```python
from build123d import *

# Parameters (mm, degrees)
SKETCH_2_R      = 27.5
SKETCH_2_R_2    = 15
SKETCH_2_R_3    = 1.5
EXTRUDE_4_DEPTH = 2


with BuildPart() as part:
    # 草图2 → 凸台-拉伸4 (new body)
    with BuildSketch(Plane.XY):
        with Locations((139.999999999, 2e-09)):
            Circle(SKETCH_2_R)
        with Locations((139.999999999, 2e-09)):
            Circle(SKETCH_2_R_2, mode=Mode.SUBTRACT)
        with Locations((156.999999999, -16.999999998)):
            Circle(SKETCH_2_R_3, mode=Mode.SUBTRACT)
        with Locations((122.999999999, -16.999999998)):
            Circle(SKETCH_2_R_3, mode=Mode.SUBTRACT)
        with Locations((122.999999999, 17.000000002)):
            Circle(SKETCH_2_R_3, mode=Mode.SUBTRACT)
        with Locations((156.999999999, 17.000000002)):
            Circle(SKETCH_2_R_3, mode=Mode.SUBTRACT)
        with Locations((149.999999999, 17.320508077)):
            Circle(SKETCH_2_R_3, mode=Mode.SUBTRACT)
        with Locations((129.917171064, 19.639898968)):
            Circle(SKETCH_2_R_3, mode=Mode.SUBTRACT)
        with Locations((129.917171064, -19.639898965)):
            Circle(SKETCH_2_R_3, mode=Mode.SUBTRACT)
        with Locations((149.999999999, -17.320508074)):
            Circle(SKETCH_2_R_3, mode=Mode.SUBTRACT)
        with Locations((157.320508075, -9.999999999)):
            Circle(SKETCH_2_R_3, mode=Mode.SUBTRACT)
        with Locations((157.320508075, 10.000000001)):
            Circle(SKETCH_2_R_3, mode=Mode.SUBTRACT)
    extrude(amount=EXTRUDE_4_DEPTH)


solid = part.part
```
Work out the finished part from the listing and answer in its coordinate system (mm). Coordinates: 2 decimals unless noted, no trailing zeros. Loops run counter-clockwise (first coordinate to the right, second up) from the corner with the lowest first, then second, coordinate; pieces in that order, holes last.
1) Consider probe 1 along Y at (x, z) = (131, 1.85); probe 2 along Y at (x, z) = (150, 0.45); probe 3 along X at (y, z) = (-13, 0.6). Determine where each line is inside the solid, lowest interval first.
Results:
probe 1: y = -25.99 to -20.68, -18.6 to -12, 12 to 18.6, 20.68 to 25.99
probe 2: y = -25.62 to -18.82, -15.82 to -11.18, 11.18 to 15.82, 18.82 to 25.62
probe 3: x = 115.77 to 132.52, 147.48 to 164.23
2) Section B-B (y = 0) is taken. Give the vertices of the cut face in (x, z), plus the area to 3 significant figures.
Results:
outline: (112.5, 0) - (125, 0) - (125, 2) - (112.5, 2) - close; (155, 0) - (167.5, 0) - (167.5, 2) - (155, 2) - close
area: 50.0 mm2
3) For a pull along Y with two mould halves and no side action, classify faces 1 (the flat face through (152, -12, 2)), 2 (the cylindrical face through (151.386, -17.895, 0.986)), 3 (the cylindrical face through (158.386, 16.425, 0.986)), 4 (the cylindrical face through (165.403, -10.533, 0.986)) as +Y half, -Y half, draft (parallel to the pull), parting line (faces both ways), or undercut.
Results:
face 1: draft
face 2: undercut
face 3: undercut
face 4: parting line
4) Section A-A (x = 140) is taken. Give the vertices of the cut face in (y, z), plus the area to 3 significant figures.
Results:
outline: (-27.5, 0) - (-15, 0) - (-15, 2) - (-27.5, 2) - close; (15, 0) - (27.5, 0) - (27.5, 2) - (15, 2) - close
area: 50.0 mm2
5) Section C-C (x = 157) is taken. Give the vertices of the cut face in (y, z).
Results:
outline: (-21.62, 0) - (-18.5, 0) - (-18.5, 2) - (-21.62, 2) - close; (-15.5, 0) - (-11.47, 0) - (-11.47, 2) - (-15.5, 2) - close; (-8.53, 0) - (8.53, 0) - (8.53, 2) - (-8.53, 2) - close; (11.47, 0) - (15.5, 0) - (15.5, 2) - (11.47, 2) - close; (18.5, 0) - (21.62, 0) - (21.62, 2) - (18.5, 2) - close
6) Section D-D (z = 1.65) is taken. Give the number of separate pieces and of enclosed holes in the cut face, plus the area to 3 significant figures.
Results:
separate pieces: 1
enclosed holes: 11
area: 1,600 mm2
7) Flat-ended cylindrical pins translate along their axes: pin 1 (2.5 mm diameter, centred on x = 150, y = -17.32, fed in from -Z); pin 2 (1 mm diameter, centred on y = 1.5, z = 0.5, fed in from +X). Find the tip coordinate at first contact, or state that the pin passes through.
Results:
pin 1: passes through
pin 2: stops at x = 167.48
